Solid Edge part; units mm, degrees
sketch "Sketch1" plane through (0, 0, 0) normal (0, 0, 1) x (1, 0, 0)
  line L0 (110, 0) -> (110, 110)
  line L1 (110, 110) -> (0, 110)
  line L2 (0, 110) -> (0, 0)
  line L3 (0, 0) -> (110, 0)
extrude "Protrusion1" add sketch "Sketch1" along normal blind 10
hole "Agujero_1" at (6, 104, 10) direction (0, 0, -1) diameter 3 end through all counterbore diameter 6 counterbore depth 3
sketch "Sketch2" plane through (55, 0, 5) normal (0, -1, 0) x (1, 0, 0)
  line L0 (5, -2.5) -> (5, 2.5)
  line L1 (5, 2.5) -> (-5, 2.5)
  line L2 (-5, 2.5) -> (-5, -2.5)
  line L3 (-5, -2.5) -> (5, -2.5)
extrude "ProtrusiónExtruida_2" add sketch "Sketch2" along normal blind 10
sketch "Sketch3" plane through (110, 55, 5) normal (1, 0, 0) x (0, 1, 0)
  line L0 (5.05, -2.55) -> (5.05, 2.55)
  line L1 (5.05, 2.55) -> (-5.05, 2.55)
  line L2 (-5.05, 2.55) -> (-5.05, -2.55)
  line L3 (-5.05, -2.55) -> (5.05, -2.55)
extrude "VaciadoExtruido_1" cut sketch "Sketch3" against normal blind 10.2
Verification items for the finished model (mm, model axes). A direction names the side the tool comes from. Round coordinates to 2 decimals unless told otherwise and drop trailing zeros. Write each loop counter-clockwise with the first axis right and the second up, starting at its lowest first coordinate (ties: lowest second). Pieces come first, ordered by that corner, then holes.
1. Section check A-A on x = 6. Enter the section's corners in (y, z), plus the area to 3 significant figures.
2. Section check D-D on x = 54.5. Enter the section's corners in (y, z), plus the area to 3 significant figures.
3. Gauge pin test, flat ends, axial feed: P1, Ø2, axis at x = 80, z = 5.5, coming from the -Y side; P2, Ø5.5, axis at y = -6, z = 4, coming from the +X side; P3, Ø8, axis at x = 56, y = -6.5, coming from the +Z side. Record the tip position at first contact, or that the pin passes through.
4. Section check B-B on z = 5.5. Enter the section's corners in (x, y).
5. Draft check along Z on faces 5 (the flat face through (55, -5, 7.5)), 6 (the flat face through (55, -10, 5)), 7 (the flat face through (99.8, 55, 5)), 8 (the flat face through (54, 56, 0)). Enter one of: +Z half, -Z half, draft (parallel to the pull), parting line (faces both ways), or undercut.
6. Section check C-C on y = 104. Enter the section's corners in (x, z).
7. Scan lines: L1, parallel to Y at x = 6, z = 4.5; L2, parallel to Y at x = 6, z = 8.1; L3, parallel to X at y = 104, z = 3.25. Record each from-to range of solid material in increasing order.
8. Access from +Z, -Z, +X, -X, +Y, -Y to the whole of each face (thin tool, end or side, straight path). Record for faces 1 (the flat face through (105, 55, 2.45)), 2 (the flat face through (55, -5, 2.5)), 3 (the flat face through (50, -5, 5)), 4 (the cylindrical face through (6, 107, 8)).
Answer:
1. outline: (0, 0) - (102.5, 0) - (102.5, 7) - (101, 7) - (101, 10) - (0, 10) - close; (105.5, 0) - (110, 0) - (110, 10) - (107, 10) - (107, 7) - (105.5, 7) - close
1. area: 1,060 mm2
2. outline: (-10, 2.5) - (0, 2.5) - (0, 0) - (110, 0) - (110, 10) - (0, 10) - (0, 7.5) - (-10, 7.5) - close
2. area: 1,150 mm2
3. P1: stops at y = 0
3. P2: stops at x = 60
3. P3: stops at z = 7.5
4. outline: (0, 0) - (50, 0) - (50, -10) - (60, -10) - (60, 0) - (110, 0) - (110, 49.95) - (99.8, 49.95) - (99.8, 60.05) - (110, 60.05) - (110, 110) - (0, 110) - close; hole circle Ø3 at (6, 104)
5. face 5: +Z half
5. face 6: draft
5. face 7: undercut
5. face 8: -Z half
6. outline: (0, 0) - (4.5, 0) - (4.5, 7) - (3, 7) - (3, 10) - (0, 10) - close; (7.5, 0) - (110, 0) - (110, 10) - (9, 10) - (9, 7) - (7.5, 7) - close
7. L1: y = 0 to 102.5, 105.5 to 110
7. L2: y = 0 to 101, 107 to 110
7. L3: x = 0 to 4.5, 7.5 to 110
8. face 1: +X
8. face 2: -Z, +X, -X, -Y
8. face 3: +Z, -Z, -X, -Y
8. face 4: +Z
